from build123d import *

# Parameters (mm, degrees)
SKETCH1_W           = 60
SKETCH1_H           = 60
BOSS_EXTRUDE1_DEPTH = 10
SKETCH2_R           = 3.96875
CUT_EXTRUDE1_DEPTH  = 44.588989435
THREAD1_PITCH       = 2
SKETCH3_R           = 3
CUT_EXTRUDE2_DEPTH  = 10


with BuildPart() as part:
    # Sketch1 → Boss-Extrude1 (new body)
    with BuildSketch(Plane.XY):
        Rectangle(SKETCH1_W, SKETCH1_H)
    extrude(amount=BOSS_EXTRUDE1_DEPTH)

    # Sketch2 → Cut-Extrude1 (cut, through all)
    with BuildSketch(Plane.XY.offset(10)):
        Circle(SKETCH2_R)
    extrude(amount=-CUT_EXTRUDE1_DEPTH, mode=Mode.SUBTRACT)

    # Thread1: the profile of Thread Profile1 profile screwed along a right-hand helix of 5 turns, 10 arcs to a turn; built about Z, then put on its axis
    thread1_z = Axis((0, 0, 0), (0, 0, 1))
    thread1_corners = [(3.96845, 0, -0.000173205), (5.05128175, 0, 0.624999997), (5.05128175, 0, 0.874999997), (3.96845, 0, 1.5001732)]
    with BuildLine(mode=Mode.PRIVATE) as thread1_profile:
        Line(thread1_corners[0], thread1_corners[1])
        Line(thread1_corners[1], thread1_corners[2])
        Line(thread1_corners[2], thread1_corners[3])
        Line(thread1_corners[3], thread1_corners[0])
    thread1_cap = Face(thread1_profile.wire())
    thread1_turn_angles = [0, 18, 36, 54, 72, 90, 108, 126, 144, 162, 180, 198, 216, 234, 252, 270, 288, 306, 324, 342, 360]
    thread1_turn_weights = [1, 0.9510565162951535, 1, 0.9510565162951535, 1, 0.9510565162951535, 1, 0.9510565162951535, 1, 0.9510565162951535, 1, 0.9510565162951535, 1, 0.9510565162951535, 1, 0.9510565162951535, 1, 0.9510565162951535, 1, 0.9510565162951535, 1]
    thread1_turn_rails = [Edge.make_bspline([Vector(p[0], p[1], 0).rotate(thread1_z, thread1_turn_angles[k]) / thread1_turn_weights[k] + Vector(0, 0, p[2] + THREAD1_PITCH * thread1_turn_angles[k] / 360) for k in range(21)], [0, 0, 0, 1, 1, 2, 2, 3, 3, 4, 4, 5, 5, 6, 6, 7, 7, 8, 8, 9, 9, 10, 10, 10], 2, thread1_turn_weights) for p in thread1_corners]
    thread1_turn_sides = [Face.make_surface_from_curves(thread1_turn_rails[p[0]], thread1_turn_rails[p[1]]) for p in [(0, 1), (1, 2), (2, 3), (3, 0)]]
    thread1 = Plane(origin=(0, 0, 10), x_dir=(-1, 0, 0), z_dir=(0, 0, -1)) * Solid(Shell([*[p.moved(Location((0, 0, THREAD1_PITCH * i))) for i in range(5) for p in thread1_turn_sides], thread1_cap, thread1_cap.rotate(thread1_z, 1800).moved(Location((0, 0, THREAD1_PITCH * 1800 / 360)))]))
    add(thread1, mode=Mode.SUBTRACT)

    # Sketch3 → Cut-Extrude2 (cut)
    with BuildSketch(Plane.XY.offset(10)):
        with Locations((15, 15)):
            Circle(SKETCH3_R)
        with Locations((-15, 15)):
            Circle(SKETCH3_R)
        with Locations((-15, -15)):
            Circle(SKETCH3_R)
        with Locations((15, -15)):
            Circle(SKETCH3_R)
    extrude(amount=-CUT_EXTRUDE2_DEPTH, mode=Mode.SUBTRACT)


solid = part.part
Could you check a few things on this model? Use its own coordinates, in mm. Give positions to 0.01 mm unless a question says otherwise; leave off trailing zeros. Order: outer loops, then holes, each group sorted by start corner. A loop starts at its lowest first (then second) coordinate and runs counter-clockwise, first axis right, second up.
Item 1: If we section it at A-A, the plane x = -15: Write out the boundary of the cut face in (y, z), plus the area to 3 significant figures.
Item 2: If we mould it in two halves opening along X, with no side actions, what happens to faces 1 (the face through (-17.4, -16.8, 5.1)), 2 (the face through (-30, 0, 5)), 3 (the face through (30, 0, 5)), 4 (the face through (-7, 0, 0))? For each: pulls with the +X half, pulls with the -X half, needs draft (parallel to the pull), parting line crosses it, or undercut.
Item 3: I'm going to push flat-ended pins straight in: pin 1 (2 mm diameter, centred on x = -19, y = 8.5, fed in from -Z); pin 2 (5 mm diameter, centred on x = -15, y = 15, fed in from -Z). Where does each tip first touch, or does it pass through?
Item 4: I need wall thicknesses on line 1 (Y direction, x = 15, z = 7.25); line 2 (Y direction, x = -12.5, z = 0.5); line 3 (Z direction, x = -2, y = 4.5). Which ranges of each line are inside material? Lowest first, please.
Values:
1. outline: (-30, 0) - (-18, 0) - (-18, 10) - (-30, 10) - close; (-12, 0) - (12, 0) - (12, 10) - (-12, 10) - close; (18, 0) - (30, 0) - (30, 10) - (18, 10) - close
1. area: 480 mm2
2. face 1: undercut
2. face 2: pulls with the -X half
2. face 3: pulls with the +X half
2. face 4: needs draft
3. pin 1: stops at z = 0
3. pin 2: passes through
4. line 1: y = -30 to -18, -12 to 12, 18 to 30
4. line 2: y = -30 to -16.66, -13.34 to 13.34, 16.66 to 30
4. line 3: z = 0 to 0.68, 1.08 to 2.68, 3.08 to 4.68, 5.08 to 6.68, 7.08 to 8.68, 9.08 to 10
